The drawing under review shows one solid part. Ordinate dimensions are in mm from its lowest x, y, z. Coordinates: 2 decimals unless noted, no trailing zeros. Write each loop counter-clockwise with the first axis right and the second up, starting at its lowest first coordinate (ties: lowest second). Pieces come first, ordered by that corner, then holes. Notation, with made-up numbers: M -12,4.5 L 6,4.5 A22 cw 6,27.5 Z; hole C 21,54.5 d8. An arc over 180 degrees is marked long. Write each question's results on one line, items separated by ' | '. Start each with the question number.
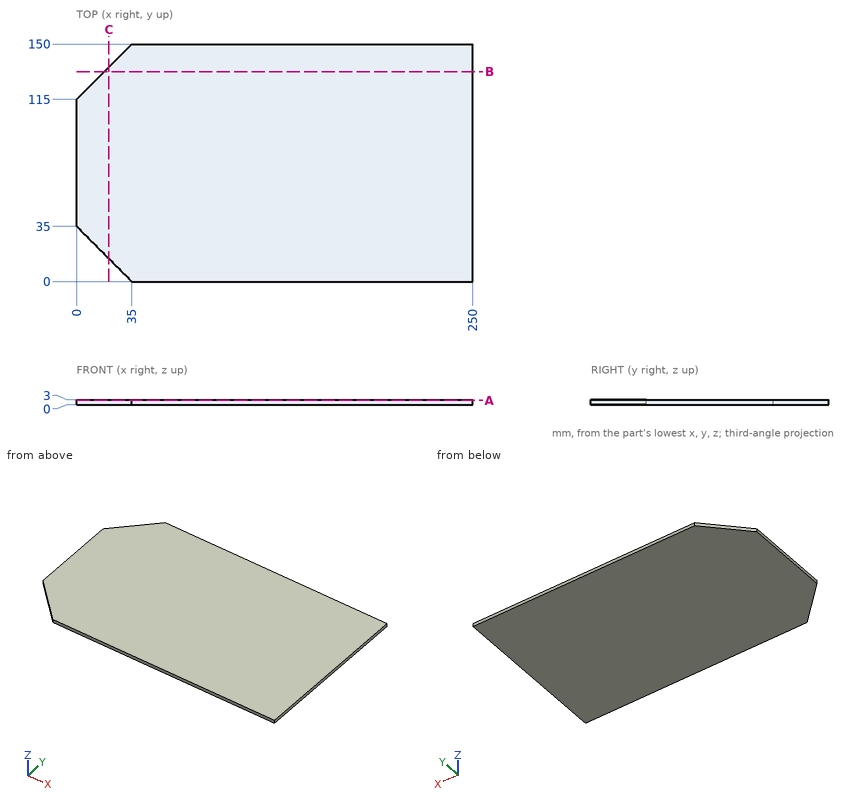
Item 1: Wall thickness on L1, parallel to X at y = 23, z = 1.2; L2, parallel to X at y = 130, z = 0.4: over which ranges is each line inside the solid? List them lowest first.
Item 2: We need section A-A on z = 2.55. State the section outline as (x, y) points, then the cut area to 3 significant figures.
Item 3: We need section C-C on x = 20.5. State the section outline as (y, z) points, then the cut area to 3 significant figures.
Item 4: We need section B-B on y = 132.5. State the section outline as (x, z) points.
Answer:
1) L1: x = 12 to 250 | L2: x = 15 to 250
2) outline: M 0,35 L 35,0 L 250,0 L 250,150 L 35,150 L 0,115 Z | area: 36,300 mm^2
3) outline: M 14.5,0 L 135.5,0 L 135.5,3 L 14.5,3 Z | area: 363 mm^2
4) outline: M 17.5,0 L 250,0 L 250,3 L 17.5,3 Z
